```python
from build123d import *

# Parameters (mm, degrees)
F1_DEPTH = 10
F3_DEPTH = 42.24330811
F4_DEPTH = 37.75869189
F6_DEPTH = 35
F7_DEPTH = 25


with BuildPart() as f1:
    # F0 (on Top) → F1 (new body)
    with BuildSketch(Plane.XY):
        Polygon((32.24230811, 22.8156701593), (-27.75769189, 22.8156701593), (-37.75769189, 12.8156701593), (-37.75769189, -37.1843298407), (42.24230811, -37.1843298407), (42.24230811, 12.8156701593), align=None)
    extrude(amount=F1_DEPTH)

    # F2 (on Right) → F3 (cut, through all)
    with BuildSketch(Plane.YZ):
        Polygon((22.8156701593, 0), (22.8156701593, 10), (12.8156701593, 10), align=None)
    extrude(amount=F3_DEPTH, mode=Mode.SUBTRACT)

    # F2 (on Right) → F4 (cut, through all)
    with BuildSketch(Plane.YZ):
        Polygon((22.8156701593, 0), (22.8156701593, 10), (12.8156701593, 10), align=None)
    extrude(amount=-F4_DEPTH, mode=Mode.SUBTRACT)

    # F5 (on Front) → F6 (cut)
    with BuildSketch(Plane.XZ):
        Polygon((37.24230811, 5), (42.24230811, 10), (-37.75769189, 10), (-32.75769189, 5), align=None)
    extrude(amount=F6_DEPTH, mode=Mode.SUBTRACT)

    # F5 (on Front) → F7 (cut)
    with BuildSketch(Plane.XZ):
        Polygon((37.24230811, 5), (42.24230811, 10), (-37.75769189, 10), (-32.75769189, 5), align=None)
    extrude(amount=-F7_DEPTH, mode=Mode.SUBTRACT)


solid = f1.part
```
For this review, take the finished solid that the model builds, in its own axes (mm). A direction names the side the tool comes from. Coordinates: 2 decimals unless noted, no trailing zeros. Order: outer loops, then holes, each group sorted by start corner. A loop starts at its lowest first (then second) coordinate and runs counter-clockwise, first axis right, second up. Notation, with made-up numbers: (-18, -27) - (-12, -27) arc R36 cw to (-12, 9) - close; hole circle Ø9 at (7.25, 64.25). An arc over 180 degrees is marked (long way). Answer as a JSON object with one key per item and string values. Group by question number.
1. For probe 1 along Z at (x, y) = (9.5, -33.5); probe 2 along Y at (x, z) = (38, 7.75); probe 3 along X at (y, z) = (-8, 7.75), list the stretches that pass through material, from the lowest coordinate up.
2. The part is to be moulded in two halves that separate along X. For faces 1 (the flat face through (-35.293, -8.962, 7.535)), 2 (the flat face through (42.242, -13, 5)), 3 (the flat face through (1.752, 20.281, 2.535)), say which applies: pulls with the +X half, pulls with the -X half, needs draft (parallel to the pull), parting line crosses it, or undercut.
3. For faces 4 (the flat face through (39.71, -8.22, 7.47)), 5 (the flat face through (2, -37.184, 5)), list the 3-axis set-ups (+Z, -Z, +X, -X, +Y, -Y) from which the entire face can be reached by the end or side of a thin tool; tool diameter is ignored.
4. We need section C-C on z = 7.75. State the section outline as (x, y) points, then the cut area to 3 significant figures.
5. We need section A-A on y = -28. State the section outline as (x, z) points.
6. We need section B-B on x = 5. State the section outline as (y, z) points, then the cut area to 3 significant figures.
7. Clearance check with flat-ended pins moving along their axes: P1, Ø2, axis at x = 22, z = 8.5, coming from the +Y side; P2, Ø5.5, axis at x = 9, z = 7.5, coming from the +Y side; P3, Ø6, axis at x = 17.5, z = 4, coming from the +Y side. State where each tip first meets the part, or that it passes through.
Final values:
{
 "1": {"probe 1": "0 to 5", "probe 2": "-37.18 to -35", "probe 3": "-37.76 to -35.51, 39.99 to 42.24"},
 "2": {"face 1": "undercut", "face 2": "pulls with the +X half", "face 3": "needs draft"},
 "3": {"face 4": "+Z, +Y", "face 5": "+Z, -Z, +X, -X, -Y"},
 "4": {"outline": "(-37.76, -37.18) - (42.24, -37.18) - (42.24, 12.82) - (39.99, 15.07) - (39.99, -35) - (-35.51, -35) - (-35.51, 15.07) - (-37.76, 12.82) - close", "area": "395 mm²"},
 "5": {"outline": "(-37.76, 0) - (42.24, 0) - (42.24, 10) - (37.24, 5) - (-32.76, 5) - (-37.76, 10) - close"},
 "6": {"outline": "(-37.18, 0) - (22.82, 0) - (17.82, 5) - (-35, 5) - (-35, 10) - (-37.18, 10) - close", "area": "298 mm²"},
 "7": {"P1": "y = -35", "P2": "y = 18.07", "P3": "y = 21.82"}
}
